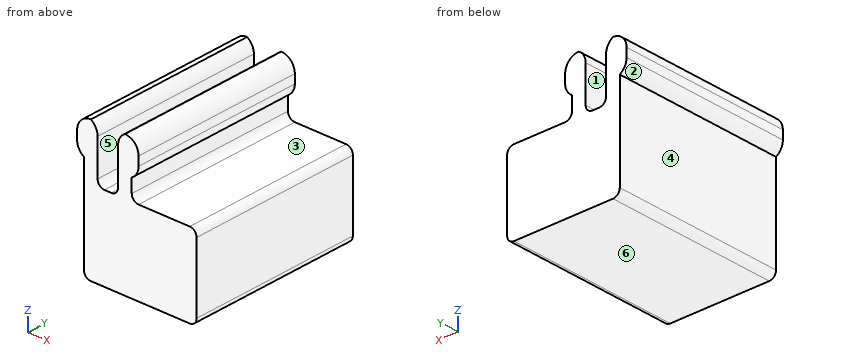
Autodesk Inventor part; units mm, degrees
ref_plane "YZ Plane" through (0, 0, 0) normal (1, 0, 0) x (0, 1, 0)
ref_plane "XZ Plane" through (0, 0, 0) normal (0, 1, 0) x (-1, 0, 0)
ref_plane "XY Plane" through (0, 0, 0) normal (0, 0, 1) x (1, 0, 0)
sketch "Sketch1" plane through (0, 0, 0) normal (0, 1, 0) x (-1, 0, 0)
  line L0 (0, 0) -> (-16.5, 0)
  line L1 (-16.5, 0) -> (-16.5, -12)
  line L2 (-16.5, -12) -> (0, -12)
  line L3 (0, -12) -> (0, 0)
  line L4 (-5, 0) -> (-7, 0)
  line L5 (-7, 0) -> (-7, 8)
  line L6 (-7, 8) -> (-5, 8)
  line L7 (-5, 8) -> (-5, 0)
  line L8 (0, 0) -> (-2, 0)
  line L9 (-2, 0) -> (-2, 8)
  line L10 (-2, 8) -> (0, 8)
  line L11 (0, 8) -> (0, 0)
  line L12 (0, 8) -> (1, 8)
  line L13 (1, 8) -> (1, 3)
  line L14 (1, 3) -> (0, 3)
  line L15 (0, 3) -> (0, 8)
  line L16 (-7, 8) -> (-8, 8)
  line L17 (-8, 8) -> (-8, 3)
  line L18 (-8, 3) -> (-7, 3)
  line L19 (-7, 3) -> (-7, 8)
  dimension "d0" = 16.5
  dimension "d1" = 12
  dimension "d4" = 2
  dimension "d5" = 8
  dimension "d6" = 3
  dimension "d9" = 1
  dimension "d10" = 5
extrude "Extrusion1" add sketch "Sketch1" along normal blind 25.4
fillet "Fillet1" radius 2 4 edges at (8, 12.7, 3) (8, 12.7, 8) (-1, 12.7, 3) (-1, 12.7, 8)
fillet "Fillet2" radius 1 3 edges at (16.5, 12.7, 0) (16.5, 12.7, -12) (0, 12.7, -12)
fillet "Fillet3" radius 1 3 edges at (5, 12.7, 0) (2, 12.7, 0) (7, 12.7, 0)
fillet "Fillet4" radius 2 2 edges at (5, 12.7, 8) (2, 12.7, 8)
properties part number "ledholder"
Read the model definition and answer for the solid it produces. Units are mm, in the model's axes. Face numbers are marked on the shaded views. A direction names the side the tool comes from. Round coordinates to 2 decimals unless told otherwise and drop trailing zeros. Write each loop counter-clockwise with the first axis right and the second up, starting at its lowest first coordinate (ties: lowest second). Pieces come first, ordered by that corner, then holes. Notation, with made-up numbers: M 50,2 L 62,2 A20 ccw 62,6 Z; hole C 82,14.5 d1. An arc over 180 degrees is marked long. One line per item, written item: value.
Q1. Find section D-D on z = -9.75. Write down the section's boundary in (x, y), plus the area to 3 significant figures.
Data:
outline: M 0,0 L 16.5,0 L 16.5,25.4 L 0,25.4 Z
area: 419 mm2
Q2. Find section C-C on x = 9. Write down the section's boundary in (y, z), plus the area to 3 significant figures.
Data:
outline: M 0,-12 L 25.4,-12 L 25.4,0 L 0,0 Z
area: 305 mm2
Q3. Find section B-B on y = 6.75. Write down the section's boundary in (x, z), plus the area to 3 significant figures.
Data:
outline: M -1,4.73 A2 ccw 0,3 L 0,-11 A1 ccw 1,-12 L 15.5,-12 A1 ccw 16.5,-11 L 16.5,-1 A1 ccw 15.5,0 L 8,0 A1 cw 7,1 L 7,3 A2 ccw 8,4.73 L 8,6 A2 ccw 6,8 A2 ccw 5,6.27 L 5,1 A1 cw 4,0 L 3,0 A1 cw 2,1 L 2,6.27 A2 ccw 1,8 A2 ccw -1,6 Z
area: 236 mm2
Q4. Find section A-A on z = 2. Write down the section's boundary in (x, y), plus the area to 3 significant figures.
Data:
outline: M 0,0 L 2,0 L 2,25.4 L 0,25.4 Z; M 5,0 L 7,0 L 7,25.4 L 5,25.4 Z
area: 102 mm2
Q5. Flat-ended cylindrical pins translate along their axes: pin 1 Ø1.6 at (y, z) = (14, 2.5) entering from +X; pin 2 Ø8 at (x, y) = (11.5, 14.5) entering from +Z; pin 3 Ø6 at (y, z) = (14, 4.5) entering from -X; pin 4 Ø1 at (x, y) = (9.5, 11.5) entering from +Z. Find the tip coordinate at first contact, or state that the pin passes through.
Data:
pin 1: x = 7.4
pin 2: z = 7.32
pin 3: x = -1
pin 4: z = 0
Q6. For a pull along X with two mould halves and no side action, classify the marked faces 4, 5 and 6 as +X half, -X half, draft (parallel to the pull), parting line (faces both ways), or undercut.
Data:
face 4: -X half
face 5: undercut
face 6: draft
Q7. Straight lines are drawn through the part: line 1 (X direction, y = 12.25, z = 5.5); line 2 (X direction, y = 23.75, z = -1.5); line 3 (Z direction, x = 10.25, y = 16). For each, find the intervals that lie inside material, in ascending order. Write a range as [from, to].
Data:
line 1: [-1, 2], [5, 8]
line 2: [0, 16.5]
line 3: [-12, 0]
Q8. Which of the six approach directions +Z, -Z, +X, -X, +Y, -Y give full straight-line access (tool end or side, diameter ignored) to the marked faces 1, 2 and 3?
Data:
face 1: +Z, +Y, -Y
face 2: -Z, -X, +Y, -Y
face 3: +Z, +X, +Y, -Y
